Geometry: final body of the model. Coordinates: model frame, mm. Coordinates: 2 decimals unless noted, no trailing zeros. Write each loop counter-clockwise with the first axis right and the second up, starting at its lowest first coordinate (ties: lowest second). Pieces come first, ordered by that corner, then holes. Notation, with made-up numbers: (33.25, 64.5) - (48.25, 64.5) arc R15 cw to (48.25, 76.5) - close; hole circle Ø1 at (33.5, 76.5). An arc over 180 degrees is marked (long way). Put each result on its own line as item: value.
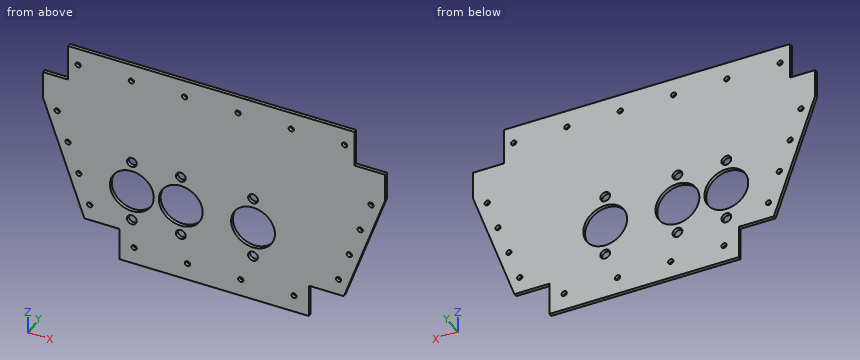
```python
from build123d import *

# Parameters (mm, degrees)
F0_R     = 2.3876
F0_R_2   = 4.445
F0_R_3   = 19.8501
F1_DEPTH = 3.175


with BuildPart() as f1:
    # F0 (on Front) → F1 (new body)
    with BuildSketch(Plane.XZ):
        Polygon((-85.725, -97.6376), (85.725, -97.6376), (85.725, -67.4624), (117.475, -67.4624), (154.94, 40.4876), (154.94, 65.8876), (126.999999, 65.8876), (126.999999, 99.341046), (-132.080001, 99.341046), (-132.080001, 65.8876), (-154.94, 65.8876), (-154.94, 40.4876), (-117.475, -67.4624), (-85.725, -67.4624), align=None)
        with Locations((-112.640408, -52.34178)):
            Circle(F0_R, mode=Mode.SUBTRACT)
        with Locations((-72.39, -81.7626)):
            Circle(F0_R, mode=Mode.SUBTRACT)
        with Locations((-24.13, -81.7626)):
            Circle(F0_R, mode=Mode.SUBTRACT)
        with Locations((-74.4728, -54.6862)):
            Circle(F0_R_2, mode=Mode.SUBTRACT)
        with Locations((-30.1752, -54.6862)):
            Circle(F0_R_2, mode=Mode.SUBTRACT)
        with Locations((-122.451709, -24.370819)):
            Circle(F0_R, mode=Mode.SUBTRACT)
        with Locations((-74.4728, -26.1112)):
            Circle(F0_R_3, mode=Mode.SUBTRACT)
        with Locations((-30.1752, -26.1112)):
            Circle(F0_R_3, mode=Mode.SUBTRACT)
        with Locations((24.13, -81.7626)):
            Circle(F0_R, mode=Mode.SUBTRACT)
        with Locations((72.39, -81.7626)):
            Circle(F0_R, mode=Mode.SUBTRACT)
        with Locations((35.2298, -54.6862)):
            Circle(F0_R_2, mode=Mode.SUBTRACT)
        with Locations((112.640408, -52.34178)):
            Circle(F0_R, mode=Mode.SUBTRACT)
        with Locations((35.2298, -26.1112)):
            Circle(F0_R_3, mode=Mode.SUBTRACT)
        with Locations((122.451709, -24.370819)):
            Circle(F0_R, mode=Mode.SUBTRACT)
        with Locations((-132.263011, 3.600143)):
            Circle(F0_R, mode=Mode.SUBTRACT)
        with Locations((-142.074312, 31.571104)):
            Circle(F0_R, mode=Mode.SUBTRACT)
        with Locations((-74.4728, 2.4638)):
            Circle(F0_R_2, mode=Mode.SUBTRACT)
        with Locations((-30.1752, 2.4638)):
            Circle(F0_R_2, mode=Mode.SUBTRACT)
        with Locations((-123.190001, 83.466046)):
            Circle(F0_R, mode=Mode.SUBTRACT)
        with Locations((-74.930001, 83.466046)):
            Circle(F0_R, mode=Mode.SUBTRACT)
        with Locations((-26.670001, 83.466046)):
            Circle(F0_R, mode=Mode.SUBTRACT)
        with Locations((35.2298, 2.4638)):
            Circle(F0_R_2, mode=Mode.SUBTRACT)
        with Locations((132.263011, 3.600143)):
            Circle(F0_R, mode=Mode.SUBTRACT)
        with Locations((142.074312, 31.571104)):
            Circle(F0_R, mode=Mode.SUBTRACT)
        with Locations((21.589999, 83.466046)):
            Circle(F0_R, mode=Mode.SUBTRACT)
        with Locations((69.849999, 83.466046)):
            Circle(F0_R, mode=Mode.SUBTRACT)
        with Locations((118.109999, 83.466046)):
            Circle(F0_R, mode=Mode.SUBTRACT)
    extrude(amount=F1_DEPTH)


solid = f1.part
```
1. Ray query, probe 1 along Z at (x, y) = (-22, -2.7); probe 2 along X at (y, z) = (-0.65, -8.5); probe 3 along X at (y, z) = (-1.35, -56.5). Return the intervals inside material, ascending. Write a range as from..to.
Answer below:
probe 1: z = -97.64..-82.84, -80.68..-44.2, -8.02..99.34
probe 2: x = -137.94..-83.63, -65.31..-39.33, -21.02..26.07, 44.39..137.94
probe 3: x = -121.28..-78.53, -70.41..-34.23, -26.12..31.17, 39.29..121.28
2. Section query B-B (z = -32). Return loops of the section in (x, y) (3 decimals).
Answer below:
outline: (-129.783, -3.175) - (-93.429, -3.175) - (-93.429, 0) - (-129.783, 0) - close; (-55.516, -3.175) - (-49.132, -3.175) - (-49.132, 0) - (-55.516, 0) - close; (-11.219, -3.175) - (16.273, -3.175) - (16.273, 0) - (-11.219, 0) - close; (54.186, -3.175) - (129.783, -3.175) - (129.783, 0) - (54.186, 0) - close
3. Section query D-D (y = -2.65). Count the separate pieces of the cut face and the enclosed holes in it, then the cut area to 3 significant figures.
Answer below:
separate pieces: 1
enclosed holes: 27
area: 46,700 mm²
4. Section query C-C (z = 10). Return loops of the section in (x, y) (3 decimals), then the cut area to 3 significant figures.
Answer below:
outline: (-144.359, -3.175) - (144.359, -3.175) - (144.359, 0) - (-144.359, 0) - close
area: 917 mm²
5. Pin query (flat end, axial travel): pin 1 Ø1 at (x, y) = (102, -1.5) entering from -Z; pin 2 Ø6 at (x, z) = (-123.19, 83.47) entering from +Y; pin 3 Ø1.5 at (y, z) = (-2, -53.5) entering from +X; pin 4 Ø1 at (y, z) = (-2.5, -54) entering from +X. Return the tip coordinate at first contact, or that it passes through.
Answer below:
pin 1: stops at z = -67.46
pin 2: stops at y = 0
pin 3: stops at x = 122.58
pin 4: stops at x = 122.32
6. Section query A-A (x = 46.5). Return loops of the section in (y, z) (3 decimals), then the cut area to 3 significant figures.
Answer below:
outline: (-3.175, -97.638) - (0, -97.638) - (0, -42.452) - (-3.175, -42.452) - close; (-3.175, -9.771) - (0, -9.771) - (0, 99.341) - (-3.175, 99.341) - close
area: 522 mm²
